Source: CAD feature listing. Evaluate the final solid. Frame: model axes, mm. Face numbers are marked on the shaded views. A direction names the side the tool comes from. Give positions to 0.01 mm unless a question says otherwise; leave off trailing zeros. Loops run counter-clockwise (first coordinate to the right, second up) from the corner with the lowest first, then second, coordinate; pieces in that order, holes last. Notation, with made-up numbers: M 84.5,71 L 95.5,71 A28 cw 95.5,100 Z; hole C 51.5,60.5 d5. An arc over 180 degrees is marked long. Answer in a Markdown table with one row per item.
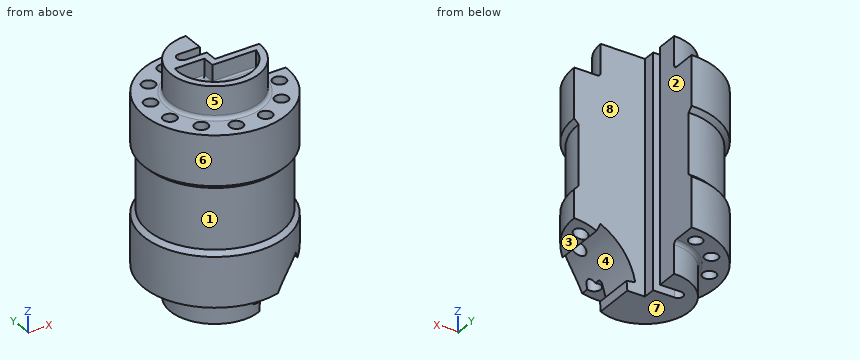
```python
from build123d import *

# Parameters (mm, degrees)
CUT_EXTRUDE1_DEPTH      = 66.5
CUT_EXTRUDE1_DEPTH_BACK = 66.5
CUT_EXTRUDE3_DEPTH      = 41
SKETCH4_R               = 3.75
CUT_EXTRUDE4_DEPTH      = 66.5000001
CUT_EXTRUDE4_DEPTH_BACK = 66.5000001
CUT_EXTRUDE5_DEPTH      = 10
FILLET1_R               = 1


with BuildPart() as part:
    # Sketch1 → Revolve1 (revolve)
    with BuildSketch(Plane(origin=(0, 0, 0), x_dir=(0, 0, -1), z_dir=(1, 0, 0))):
        with BuildLine():
            Line((65.5, 0), (-65.5, 0))
            Line((-65.5, 0), (-65.5, 25))
            Line((-65.5, 25), (-49.5, 25))
            ThreePointArc((-49.5, 25), (-48.085786438, 25.585786438), (-47.5, 27))
            Line((-47.5, 27), (-47.5, 40))
            Line((-47.5, 40), (-19.5, 40))
            Line((-19.5, 40), (-17, 37.5))
            Line((-17, 37.5), (17, 37.5))
            Line((17, 37.5), (19.5, 40))
            Line((19.5, 40), (47.5, 40))
            Line((47.5, 40), (47.5, 27))
            ThreePointArc((47.5, 27), (48.085786438, 25.585786438), (49.5, 25))
            Line((49.5, 25), (65.5, 25))
            Line((65.5, 25), (65.5, 0))
        make_face()
    revolve(axis=Axis((0, 0, -65.5), (0, 0, 1)))

    # Sketch2 → Cut-Extrude1 (cut, two sides)
    with BuildSketch(Plane.XY) as cut_extrude1_sk:
        with BuildLine():
            Line((0, 40), (0, 13))
            Line((0, 13), (-12, 13))
            ThreePointArc((-12, 13), (-15, 10), (-12, 7))
            Line((-12, 7), (0, 7))
            Line((0, 7), (0, 0))
            Line((0, 0), (40, 0))
            ThreePointArc((40, 0), (28.284271247, 28.284271247), (0, 40))
        make_face()
    extrude(amount=CUT_EXTRUDE1_DEPTH, mode=Mode.SUBTRACT)
    extrude(cut_extrude1_sk.sketch, amount=-CUT_EXTRUDE1_DEPTH_BACK, mode=Mode.SUBTRACT)

    # Sketch3 → Cut-Extrude3 (cut, through all)
    with BuildSketch(Plane(origin=(0, 0, 0), x_dir=(1, 0, 0), z_dir=(0, 1, 0))):
        with BuildLine():
            Line((27.321452148, 38.310766389), (25.208360839, 33.779227454))
            ThreePointArc((25.208360839, 33.779227454), (12.23263309, 44.193349985), (5.531728645, 59.422313782))
            Line((5.531728645, 59.422313782), (10.45576741, 60.29055467))
            ThreePointArc((10.45576741, 60.29055467), (63.800600209, 83.76284287), (27.321452148, 38.310766389))
        make_face()
    extrude(amount=-CUT_EXTRUDE3_DEPTH, mode=Mode.SUBTRACT)

    # Sketch4 → Cut-Extrude4 (cut, two sides)
    with BuildSketch(Plane.XY) as cut_extrude4_sk:
        with Locations((-8.282209443, 30.909626441)):
            Circle(SKETCH4_R)
        with Locations((8.282209443, 30.909626441)):
            Circle(SKETCH4_R)
        with Locations((22.627416998, 22.627416998)):
            Circle(SKETCH4_R)
        with Locations((30.909626441, 8.282209443)):
            Circle(SKETCH4_R)
        with Locations((30.909626441, -8.282209443)):
            Circle(SKETCH4_R)
        with Locations((22.627416998, -22.627416998)):
            Circle(SKETCH4_R)
        with Locations((8.282209443, -30.909626441)):
            Circle(SKETCH4_R)
        with Locations((-8.282209443, -30.909626441)):
            Circle(SKETCH4_R)
        with Locations((-22.627416998, -22.627416998)):
            Circle(SKETCH4_R)
        with Locations((-30.909626441, -8.282209443)):
            Circle(SKETCH4_R)
        with Locations((-30.909626441, 8.282209443)):
            Circle(SKETCH4_R)
        with Locations((-22.627416998, 22.627416998)):
            Circle(SKETCH4_R)
    extrude(amount=CUT_EXTRUDE4_DEPTH, mode=Mode.SUBTRACT)
    extrude(cut_extrude4_sk.sketch, amount=-CUT_EXTRUDE4_DEPTH_BACK, mode=Mode.SUBTRACT)

    # Sketch5 → Cut-Extrude5 (cut)
    with BuildSketch(Plane.XY.offset(65.5)):
        with BuildLine():
            Line((-20.784609691, 3), (-4, 3))
            Line((-4, 3), (-4, -4))
            Line((-4, -4), (20.615528128, -4))
            ThreePointArc((20.615528128, -4), (-3.501020872, -20.706106656), (-20.784609691, 3))
        make_face()
    extrude(amount=-CUT_EXTRUDE5_DEPTH, mode=Mode.SUBTRACT)

    # Fillet1
    fillet1_edges = [part.edges().sort_by_distance(p)[0] for p in [
        (-3.501020872, -20.706106656, 55.5),
        (-12.392304845, 3, 55.5),
        (-4, -0.5, 55.5),
        (8.307764064, -4, 55.5),
    ]]
    fillet(fillet1_edges, radius=FILLET1_R)


solid = part.part
```
1) Pin query (flat end, axial travel): pin 1 Ø5 at (y, z) = (-22, 2.5) entering from +X; pin 2 Ø4 at (y, z) = (-19.5, 14) entering from -X; pin 3 Ø4 at (x, z) = (25.5, -38.5) entering from +Y. Return the tip coordinate at first contact, or that it passes through.
Reply:
| item | result |
|---|---|
| pin 1 | stops at x = 32.03 |
| pin 2 | stops at x = -33.17 |
| pin 3 | stops at y = 0 |
2) Set-up query: the marked faces 4, 5, 6, 7 and 8. Return all of +Z, -Z, +X, -X, +Y, -Y with unobstructed straight access to the full face (end or side cutting, diameter ignored); none if empty.
Reply:
| item | result |
|---|---|
| face 4 | +Y, -Y |
| face 5 | +Z |
| face 6 | +Z, -Z |
| face 7 | -Z, +X, -X, +Y, -Y |
| face 8 | +Z, -Z, +X, +Y |
3) Section A-A, the plane z = 11. Count the separate pieces of the cut face and the enclosed holes in it, then the cut area to 3 significant figures.
Reply:
| item | result |
|---|---|
| separate pieces | 1 |
| enclosed holes | 9 |
| area | 2,830 mm² |
4) Section B-B, the plane z = -43. Return loops of the section in (x, y), then the cut area to 3 significant figures.
Reply:
| item | result |
|---|---|
| outline | M -12,7 A3 cw -12,13 L 0,13 L 0,40 A40 ccw long 13.19,-37.76 L 13.19,0 L 0,0 L 0,7 Z; hole C -30.91,-8.28 d7.5; hole C -30.91,8.28 d7.5; hole C -22.63,-22.63 d7.5; hole C -22.63,22.63 d7.5; hole C -8.28,-30.91 d7.5; hole C -8.28,30.91 d7.5; hole C 8.28,-30.91 d7.5 |
| area | 2,640 mm² |
5) Material intervals for L1, parallel to Z at x = -30, y = 3.5; L2, parallel to Y at x = -0.5, z = 5.5; L3, parallel to X at y = 31, z = -9.5, sorted ascending.
Reply:
| item | result |
|---|---|
| L1 | z = -47.5 to 47.5 |
| L2 | y = -37.5 to 7, 13 to 37.5 |
| L3 | x = -21.1 to -12.03, -4.53 to 0 |
6) Pull-direction query (Z, two-part tool) for the marked faces 1, 2 and 3; classes: released by +Z, released by -Z, zero draft, split by the parting line, or undercut.
Reply:
| item | result |
|---|---|
| face 1 | undercut |
| face 2 | zero draft |
| face 3 | released by -Z |
